from build123d import *

# Parameters (mm, degrees)
SKETCH_1_R          = 3
SKETCH_1_R_2        = 1.45
SKETCH_1_W          = 72
SKETCH_1_H          = 125
SKETCH_1_W_2        = 45
SKETCH_1_H_2        = 92.5
EXTRUDE_1_DEPTH     = 5
SKETCH_2_W          = 5
SKETCH_2_H          = 13
CUT_EXTRUDE_1_DEPTH = 215.767315949
CUT_EXTRUDE_START   = -5
SKETCH_3_W          = 12
SKETCH_3_H          = 3
CUT_EXTRUDE_2_DEPTH = 2
EXTRUDE_2_DEPTH     = 5
FILLET_1_R          = 5
FILLET_2_R          = 3
SKETCH_5_R          = 1.45
CUT_EXTRUDE_3_DEPTH = 215.767315949
EXTRUDE_START       = 5
SKETCH_6_R          = 4.45
SKETCH_6_R_2        = 1.45
EXTRUDE_3_DEPTH     = 5
SKETCH_7_W          = 5
SKETCH_7_H          = 20
EXTRUDE_4_DEPTH     = 5
SKETCH_8_R          = 1.45
CUT_EXTRUDE_4_DEPTH = 217.275842387
FILLET_3_R          = 3
SKETCH_9_R          = 1
CUT_EXTRUDE_5_DEPTH = 217.275842387
FILLET_4_R          = 1
FILLET_5_R          = 1
SKETCH_10_W         = 11
SKETCH_10_H         = 20
CUT_EXTRUDE_6_DEPTH = 10
FILLET_6_R          = 2


with BuildPart() as part:
    # 草图1 → 凸台-拉伸1 (new body)
    with BuildSketch(Plane.XY):
        Polygon((-57, 190), (-57, 20), (0, 20), (0, 0), (100, 0), (100, 155), (15, 155), (15, 190), align=None)
        with Locations((-45, 175)):
            Circle(SKETCH_1_R, mode=Mode.SUBTRACT)
        with Locations((-1, 175)):
            Circle(SKETCH_1_R, mode=Mode.SUBTRACT)
        with Locations((-1, 32.5)):
            Circle(SKETCH_1_R, mode=Mode.SUBTRACT)
        with Locations((-45, 32.5)):
            Circle(SKETCH_1_R, mode=Mode.SUBTRACT)
        with Locations((30, 7.5)):
            Circle(SKETCH_1_R_2, mode=Mode.SUBTRACT)
        with Locations((50, 7.5)):
            Circle(SKETCH_1_R_2, mode=Mode.SUBTRACT)
        with Locations((30, 147.5)):
            Circle(SKETCH_1_R_2, mode=Mode.SUBTRACT)
        with Locations((50, 147.5)):
            Circle(SKETCH_1_R_2, mode=Mode.SUBTRACT)
        with Locations((70, 147.5)):
            Circle(SKETCH_1_R_2, mode=Mode.SUBTRACT)
        with Locations((70, 7.5)):
            Circle(SKETCH_1_R_2, mode=Mode.SUBTRACT)
        with Locations((56, 77.5)):
            Rectangle(SKETCH_1_W, SKETCH_1_H, mode=Mode.SUBTRACT)
        with Locations((-22.5, 108.75)):
            Rectangle(SKETCH_1_W_2, SKETCH_1_H_2, mode=Mode.SUBTRACT)
    extrude(amount=EXTRUDE_1_DEPTH)

    # 草图2 → 切除-拉伸1 (cut, through all)
    with BuildSketch(Plane.XY.offset(5)):
        with Locations((-23, 171)):
            Rectangle(SKETCH_2_W, SKETCH_2_H)
        with Locations((-23, 50.5)):
            Rectangle(SKETCH_2_W, SKETCH_2_H)
    extrude(amount=-CUT_EXTRUDE_1_DEPTH, mode=Mode.SUBTRACT)

    # 草图3 → 切除-拉伸2 (cut)
    with BuildSketch(Plane.XY.offset(5).offset(CUT_EXTRUDE_START)):
        with Locations((-23, 50.5)):
            Rectangle(SKETCH_3_W, SKETCH_3_H)
        with Locations((-23, 171)):
            Rectangle(SKETCH_3_W, SKETCH_3_H)
    extrude(amount=CUT_EXTRUDE_2_DEPTH, mode=Mode.SUBTRACT)

    # 草图4 → 凸台-拉伸2 (add)
    with BuildSketch(Plane.XY):
        Polygon((-4.523420353, 155), (-45, 67.023420353), (-45, 62.5), (-40.476579647, 62.5), (0, 150.476579647), (0, 155), align=None)
        Polygon((20, 140), (20, 132.636069246), (84.636069246, 15), (92, 15), (92, 22.363930754), (27.363930754, 140), align=None)
        Polygon((15, 190), (57.5, 155), (48.061693338, 155), (15, 182.227276866), align=None)
    extrude(amount=EXTRUDE_2_DEPTH)

    # 圆角1
    fillet_1_edges = [part.edges().sort_by_distance(p)[0] for p in [
        (15, 155, 2.5),
        (-4.523420353, 155, 2.5),
        (-45, 67.023420353, 2.5),
        (-40.476579647, 62.5, 2.5),
        (0, 150.476579647, 2.5),
        (27.363930754, 140, 2.5),
        (20, 132.636069246, 2.5),
        (84.636069246, 15, 2.5),
        (92, 22.363930754, 2.5),
        (15, 182.227276866, 2.5),
        (48.061693338, 155, 2.5),
        (20, 15, 2.5),
        (92, 140, 2.5),
        (-45, 155, 2.5),
        (0, 62.5, 2.5),
    ]]
    fillet(fillet_1_edges, radius=FILLET_1_R)

    # 圆角2
    fillet_2_edges = [part.edges().sort_by_distance(p)[0] for p in [
        (15, 190, 2.5),
        (100, 155, 2.5),
        (100, 0, 2.5),
        (0, 0, 2.5),
        (0, 20, 2.5),
        (-57, 20, 2.5),
        (-57, 190, 2.5),
        (57.5, 155, 2.5),
    ]]
    fillet(fillet_2_edges, radius=FILLET_2_R)

    # 草图5 → 切除-拉伸3 (cut, through all)
    with BuildSketch(Plane.XY.offset(5)):
        with Locations((98.75, 112.25)):
            Circle(SKETCH_5_R)
        with Locations((98.75, 62.75)):
            Circle(SKETCH_5_R)
        with Locations((33.25, 112.25)):
            Circle(SKETCH_5_R)
        with Locations((33.25, 62.75)):
            Circle(SKETCH_5_R)
    extrude(amount=-CUT_EXTRUDE_3_DEPTH, mode=Mode.SUBTRACT)

    # 草图6 → 凸台-拉伸3 (add)
    # profile 1 of 4: a face of its own
    with BuildSketch(Plane.XY.offset(EXTRUDE_START)):
        with Locations((33.25, 112.25)):
            Circle(SKETCH_6_R)
        with Locations((33.25, 112.25)):
            Circle(SKETCH_6_R_2, mode=Mode.SUBTRACT)
    # profile 2 of 4: a face of its own
    with BuildSketch(Plane.XY.offset(EXTRUDE_START)):
        with Locations((98.75, 62.75)):
            Circle(SKETCH_6_R)
        with Locations((98.75, 62.75)):
            Circle(SKETCH_6_R_2, mode=Mode.SUBTRACT)
    # profile 3 of 4: a face of its own
    with BuildSketch(Plane.XY.offset(EXTRUDE_START)):
        with Locations((98.75, 112.25)):
            Circle(SKETCH_6_R)
        with Locations((98.75, 112.25)):
            Circle(SKETCH_6_R_2, mode=Mode.SUBTRACT)
    # profile 4 of 4: a face of its own
    with BuildSketch(Plane.XY.offset(EXTRUDE_START)):
        with BuildLine():
            Line((33.25, 67.2), (20, 67.2))
            Line((20, 67.2), (20, 58.3))
            Line((20, 58.3), (33.25, 58.3))
            ThreePointArc((33.25, 58.3), (37.7, 62.75), (33.25, 67.2))
        make_face()
        with Locations((33.25, 62.75)):
            Circle(SKETCH_6_R_2, mode=Mode.SUBTRACT)
    extrude(amount=-EXTRUDE_3_DEPTH)

    # 草图7 → 凸台-拉伸4 (add)
    with BuildSketch(Plane.XY):
        with Locations((-2.5, 107.5)):
            Rectangle(SKETCH_7_W, SKETCH_7_H)
    extrude(amount=EXTRUDE_4_DEPTH)

    # 草图8 → 切除-拉伸4 (cut, through all)
    with BuildSketch(Plane.XY.offset(5)):
        with Locations((4, 117.5)):
            Circle(SKETCH_8_R)
        with Locations((4, 107.5)):
            Circle(SKETCH_8_R)
    extrude(amount=-CUT_EXTRUDE_4_DEPTH, mode=Mode.SUBTRACT)

    # 圆角3
    fillet_3_edges = [part.edges().sort_by_distance(p)[0] for p in [
        (20, 58.3, 2.5),
        (20, 67.2, 2.5),
    ]]
    fillet(fillet_3_edges, radius=FILLET_3_R)

    # 草图9 → 切除-拉伸5 (cut, through all)
    with BuildSketch(Plane.XY.offset(5)):
        with Locations((0, 117.5)):
            Circle(SKETCH_9_R)
        with Locations((0, 97.5)):
            Circle(SKETCH_9_R)
    extrude(amount=-CUT_EXTRUDE_5_DEPTH, mode=Mode.SUBTRACT)

    # 圆角4
    fillet_4_edges = [part.edges().sort_by_distance(p)[0] for p in [
        (-5, 117.5, 2.5),
        (-5, 97.5, 2.5),
    ]]
    fillet(fillet_4_edges, radius=FILLET_4_R)

    # 圆角5
    fillet_5_edges = [part.edges().sort_by_distance(p)[0] for p in [
        (-25.5, 177.5, 2.5),
        (-20.5, 177.5, 2.5),
        (-20.5, 164.5, 2.5),
        (-25.5, 164.5, 2.5),
        (-20.5, 44, 2.5),
        (-25.5, 44, 2.5),
        (-25.5, 57, 2.5),
        (-20.5, 57, 2.5),
        (-29, 49, 1),
        (-17, 49, 1),
        (-17, 52, 1),
        (-29, 52, 1),
        (-17, 172.5, 1),
        (-29, 169.5, 1),
        (-17, 169.5, 1),
        (-29, 172.5, 1),
    ]]
    fillet(fillet_5_edges, radius=FILLET_5_R)

    # 草图10 → 切除-拉伸6 (cut)
    with BuildSketch(Plane.XY.offset(5)):
        with Locations((-23, 30)):
            Rectangle(SKETCH_10_W, SKETCH_10_H)
    extrude(amount=-CUT_EXTRUDE_6_DEPTH, mode=Mode.SUBTRACT)

    # 圆角6
    fillet_6_edges = [part.edges().sort_by_distance(p)[0] for p in [
        (100, 116.520831301, 2.5),
        (100, 107.979168699, 2.5),
        (100, 58.479168699, 2.5),
        (100, 67.020831301, 2.5),
        (-17.5, 20, 2.5),
        (-28.5, 20, 2.5),
        (-28.5, 40, 2.5),
        (-17.5, 40, 2.5),
    ]]
    fillet(fillet_6_edges, radius=FILLET_6_R)


solid = part.part
Here's how the part is built. I have some questions about the finished solid (model axes, mm). A direction names the side the tool comes from. Give positions to 0.01 mm unless a question says otherwise; leave off trailing zeros. Loops run counter-clockwise (first coordinate to the right, second up) from the corner with the lowest first, then second, coordinate; pieces in that order, holes last. Notation, with made-up numbers: (-31, 53.5) -> (15, 53.5) arc R20 cw to (15, 73.5) -> close; hole circle Ø8 at (-22.5, -11.75). An arc over 180 degrees is marked (long way). One line per item, written item: value.
Q1. Suppose I cut it at B-B on z = 1. State how many separate pieces and enclosed holes the cut face has, then the cut area to 3 significant figures.
Answers follow:
separate pieces: 1
enclosed holes: 23
area: 15,000 mm^2
Q2. Suppose I cut it at A-A on y = 137.5. Please give me the cut outline in (x, z).
Answers follow:
outline: (-57, 0) -> (-45, 0) -> (-45, 5) -> (-57, 5) -> close; (-12.57, 0) -> (31.49, 0) -> (31.49, 5) -> (-12.57, 5) -> close; (91.33, 0) -> (100, 0) -> (100, 5) -> (91.33, 5) -> close
Q3. On a 3-axis mill with a long thin cutter (end or side, diameter ignored), from which of +Z, -Z, +X, -X, +Y, -Y can I reach the whole of each face in a straight line? I mean faces 4 (the face through (-9, 20, 2)), 5 (the face through (-17.5, 30, 3)), 6 (the face through (-25.5, 171, 3)), 7 (the face through (4, 96, 0)). Say none if no direction works.
Answers follow:
face 4: +Z, -Z, -X, -Y
face 5: +Z, -Z, -Y
face 6: +Z, -Z
face 7: -Z, +X, -X, +Y, -Y
Q4. If I drill on line 1 along Y through (x, z) = (-9, 1.4); line 2 along X through (y, z) = (175, 3.5); line 3 along Y through (x, z) = (50, 2.3), over which ranges is the centre line in solid material (lowest first)?
Answers follow:
line 1: 20 to 62.5, 130.65 to 145.27, 153.73 to 190
line 2: -57 to -48, -42 to -25.5, -20.5 to -4, 2 to 16.3, 23.78 to 33.21
line 3: 0 to 6.05, 8.95 to 15, 78.04 to 98.8, 140 to 146.05, 148.95 to 161.18
Q5. I'm going to push flat-ended pins straight in: pin 1 Ø3.5 at (x, y) = (33.25, 112.25) entering from +Z; pin 2 Ø1.5 at (x, y) = (-27.5, 50.5) entering from -Z; pin 3 Ø5.5 at (x, y) = (-45, 175) entering from -Z; pin 4 Ø2.5 at (y, z) = (132.5, 2) entering from +X. Where does each tip first touch, or does it pass through?
Answers follow:
pin 1: z = 5
pin 2: z = 2
pin 3: through
pin 4: x = 100
Q6. We'd pull the mould along Y, two halves only. Please class faces 1 (the face through (100, 135, 2)), 2 (the face through (-23, 40, 3)), 3 (the face through (-19, 62.5, 2)): pulls with the +Y half, pulls with the -Y half, needs draft (parallel to the pull), parting line crosses it, or undercut.
Answers follow:
face 1: needs draft
face 2: pulls with the -Y half
face 3: undercut
